Work out the finished part from the listing and answer in its coordinate system (mm). Face numbers are marked on the shaded views. A direction names the side the tool comes from. Round coordinates to 2 decimals unless told otherwise and drop trailing zeros. Write each loop counter-clockwise with the first axis right and the second up, starting at its lowest first coordinate (ties: lowest second). Pieces come first, ordered by that corner, then holes. Notation, with made-up numbers: M 67,-2.5 L 115,-2.5 A22 cw 115,16.5 Z; hole C 67.25,0.5 d3. An arc over 180 degrees is marked long. Answer in a Markdown table with one row per item.
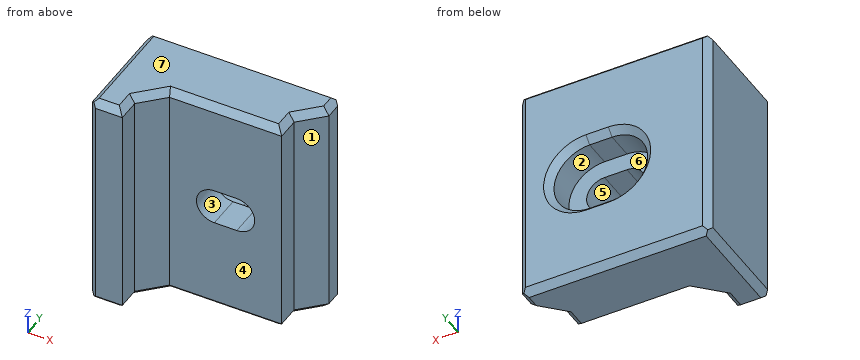
Autodesk Inventor part; units mm, degrees
ref_plane "YZ Plane" through (0, 0, 0) normal (1, 0, 0) x (0, 1, 0)
ref_plane "XZ Plane" through (0, 0, 0) normal (0, 1, 0) x (-1, 0, 0)
ref_plane "XY Plane" through (0, 0, 0) normal (0, 0, 1) x (1, 0, 0)
sketch "Sketch1" plane through (0, 0, 0) normal (0, 0, 1) x (1, 0, 0)
  line L0 (0, 0) -> (3, 0)
  line L1 (3, 0) -> (3, 2)
  line L2 (3, 2) -> (5, 4)
  line L3 (5, 4) -> (15, 4)
  line L4 (17, 10) -> (0, 10)
  line L5 (0, 10) -> (0, 0)
  line L6 (15, 4) -> (15, 6)
  line L7 (15, 6) -> (17, 8)
  line L8 (17, 8) -> (17, 10)
  dimension "d0" = 45
  dimension "d2" = 3
  dimension "d4" = 10
  dimension "d6" = 2
  dimension "d7" = 2
  dimension "d8" = 2
  dimension "d25" = 2
extrude "Extrusion1" add sketch "Sketch1" along normal blind 20
sketch "Sketch2" plane through (0, 10, 0) normal (0, 1, 0) x (1, 0, 0)
  line L0 (7.4, -10) -> (12.6, -10) construction
  line L1 (9, -11.6) -> (11, -11.6)
  line L2 (11, -8.4) -> (9, -8.4)
  arc A0 (9, -8.4) -> (9, -11.6) centre (9, -10) ccw
  arc A1 (11, -11.6) -> (11, -8.4) centre (11, -10) ccw
  line L3 (9, -10) -> (11, -10) construction
  line L4 (9, -13.175) -> (11, -13.175)
  line L5 (11, -6.825) -> (9, -6.825)
  arc A2 (9, -6.825) -> (9, -13.175) centre (9, -10) ccw
  arc A3 (11, -13.175) -> (11, -6.825) centre (11, -10) ccw
  line L6 (5, 0) -> (15, 0) construction
  line L7 (15, 0) -> (15, -20) construction
  line L8 (5, -20) -> (15, -20) construction
  line L9 (5, 0) -> (5, -20) construction
  point P0 (10, -10)
  point P1 (7.4, -10)
  point P2 (12.6, -10)
  point P3 (5.825, -10)
  point P4 (10, -20)
  point P5 (5, -10)
  dimension "d11" = 3.2
  dimension "d16" = 6.35
  dimension "d24" = 2
extrude "Extrusion2" cut sketch "Sketch2" against normal through all contours A0 L2 A1 L1
extrude "Extrusion3" cut sketch "Sketch2" against normal blind 3 contours A0 L2 A1 L1 | A2 L5 A3 L4
chamfer "Chamfer1" distance 0.6 angle 45 25 edges at (8.5, 10, 20) (8.5, 10, 0) (0, 10, 10) (0, 5, 20) (0, 5, 0) (0, 0, 10) (1.5, 0, 20) (1.5, 0, 0) (16, 7, 20) (15, 5, 20) (10, 4, 20) (4, 3, 20) (3, 1, 20) (3, 1, 0) (4, 3, 0) (10, 4, 0) (15, 5, 0) (16, 7, 0) (14.175, 10, 10) (10, 10, 13.175) (5.825, 10, 10) (10, 10, 6.825) (17, 9, 20) (17, 9, 0) (17, 10, 10)
equation "\"d7\" = d6"
equation "\"d8\" = d7"
equation "\"d25\" = d7"
1. The part is cut by section D-D (x = 15.5). Determine the outline of the cut face in (y, z), plus the area to 3 significant figures.
Calculated:
| item | result |
|---|---|
| outline | M 6.5,0.6 L 7.35,0 L 9.4,0 L 10,0.6 L 10,19.4 L 9.4,20 L 7.35,20 L 6.5,19.4 Z |
| area | 69.1 mm² |
2. A tool of negligible diameter and unlimited length cuts with its end or side. For the marked faces 5, 6 and 7, from which of +Z, -Z, +X, -X, +Y, -Y can it reach the whole face along a straight path? Write none if from no direction.
Calculated:
| item | result |
|---|---|
| face 5 | +Y, -Y |
| face 6 | +Y |
| face 7 | +Z, +X, -X, +Y, -Y |
3. The part is cut by section C-C (z = 15.75). Determine the outline of the cut face in (x, y), plus the area to 3 significant figures.
Calculated:
| item | result |
|---|---|
| outline | M 0,0.6 L 0.6,0 L 3,0 L 3,2 L 5,4 L 15,4 L 15,6 L 17,8 L 17,9.4 L 16.4,10 L 0.6,10 L 0,9.4 Z |
| area | 109 mm² |
4. The part is cut by section A-A (z = 10). Determine the outline of the cut face in (x, y) (3 decimals), plus the area to 4 significant figures.
Calculated:
| item | result |
|---|---|
| outline | M 0,0.6 L 0.6,0 L 3,0 L 3,2 L 5,4 L 7.4,4 L 7.4,7 L 5.825,7 L 5.825,9.4 L 5.225,10 L 0.6,10 L 0,9.4 Z; M 12.6,4 L 15,4 L 15,6 L 17,8 L 17,9.4 L 16.4,10 L 14.775,10 L 14.175,9.4 L 14.175,7 L 12.6,7 Z |
| area | 68.45 mm² |
5. Determine the mould class of the marked faces 1, 2, 3 and 4 for opening direction X: released by +X, released by -X, zero draft, split by the parting line, or undercut.
Calculated:
| item | result |
|---|---|
| face 1 | released by +X |
| face 2 | undercut |
| face 3 | undercut |
| face 4 | zero draft |
6. Given pin 1 (0.6 mm diameter, centred on y = 5, z = 12, fed in from +X); pin 2 (3 mm diameter, centred on x = 8, z = 11, fed in from -Y); pin 3 (4 mm diameter, centred on x = 11.5, y = 5, fed in from -Z); pin 4 (3 mm diameter, centred on x = 14, y = 1.5, fed in from -Z), each flat-ended and moving along its own axis, determine where each tip first touches the part or whether it passes through.
Calculated:
| item | result |
|---|---|
| pin 1 | stops at x = 15 |
| pin 2 | stops at y = 4 |
| pin 3 | stops at z = 0 |
| pin 4 | passes through |
7. Consider line 1 along Z through (x, y) = (10.25, 5.75); line 2 along Y through (x, z) = (7, 11.75); line 3 along Y through (x, z) = (13, 3). Determine where each line is inside the solid, lowest interval first. Write a range as from..to.
Calculated:
| item | result |
|---|---|
| line 1 | z = 0..8.4, 11.6..20 |
| line 2 | y = 4..7 |
| line 3 | y = 4..10 |
8. The part is cut by section B-B (x = 9.5). Determine the outline of the cut face in (y, z) (3 decimals).
Calculated:
| item | result |
|---|---|
| outline | M 4,0.6 L 4.6,0 L 9.4,0 L 10,0.6 L 10,6.225 L 9.4,6.825 L 7,6.825 L 7,8.4 L 4,8.4 Z; M 4,11.6 L 7,11.6 L 7,13.175 L 9.4,13.175 L 10,13.775 L 10,19.4 L 9.4,20 L 4.6,20 L 4,19.4 Z |
